Here's how the part is built. I have some questions about the finished solid (model axes, mm). Give positions to 0.01 mm unless a question says otherwise; leave off trailing zeros. Loops run counter-clockwise (first coordinate to the right, second up) from the corner with the lowest first, then second, coordinate; pieces in that order, holes last. Notation, with made-up numbers: (-22.5, 83) -> (35.5, 83) arc R21 ccw to (35.5, 92) -> close; hole circle Ø11 at (66, 21.5). An arc over 180 degrees is marked (long way). Answer in a Markdown table with one row per item. Add a question column.
Item 1: For P1, Ø4, axis at x = 18, z = 11, coming from the -Y side, with a flat end and sliding along its axis, tell me the tip position at first contact or that it passes through.
Item 2: If we section it at B-B (z = 45): Write out the boundary of the cut face in (x, y).
Item 3: If I drill on line 1 (Z direction, x = 35, y = 1.3); line 2 (Z direction, x = -34.5, y = 0.9); line 3 (X direction, y = 0.75, z = 46), over which ranges is the centre line in solid material (lowest first)?
Item 4: If we section it at A-A (x = -35): Write out the boundary of the cut face in (y, z).
Item 5: We'd pull the mould along X, two halves only. Please class faces 1 (the face through (-34.675, 0.789, -43.536)), 2 (the face through (1, 0, 1)): released by +X, released by -X, zero draft, split by the parting line, or undercut.
Autodesk Inventor part; units mm, degrees
ref_plane "YZ Plane" through (0, 0, 0) normal (1, 0, 0) x (0, 1, 0)
ref_plane "XZ Plane" through (0, 0, 0) normal (0, 1, 0) x (-1, 0, 0)
ref_plane "XY Plane" through (0, 0, 0) normal (0, 0, 1) x (1, 0, 0)
sketch "Skizze1" plane through (0, 0, 0) normal (0, 1, 0) x (-1, 0, 0)
  line L0 (40, 50) -> (-40, 50)
  line L1 (-40, 50) -> (-40, -50)
  line L2 (-40, -50) -> (40, -50)
  line L3 (40, -50) -> (40, 50)
  line L4 (0, 0) -> (0, -50) construction
  line L5 (0, 0) -> (40, 0) construction
  line L6 (35, 45) -> (-35, 45) construction
  line L7 (-35, 45) -> (-35, -45) construction
  line L8 (-35, -45) -> (35, -45) construction
  line L9 (35, -45) -> (35, 45) construction
  circle A0 centre (35, 45) radius 1.5
  circle A1 centre (-35, 45) radius 1.5
  circle A2 centre (-35, -45) radius 1.5
  circle A3 centre (35, -45) radius 1.5
  point P0 (35, 0)
  point P1 (0, -45)
  dimension "d0" = 100
  dimension "d1" = 80
  dimension "d2" = 5
  dimension "d3" = 5
  dimension "d4" = 3
  dimension "d5" = 3
  dimension "d6" = 3
  dimension "d7" = 3
extrude "Extrusion1" add sketch "Skizze1" along normal blind 1.6
properties part number "Platine_MCU"
Recorded:
| question | item | result |
|---|---|---|
| 1 | P1 | stops at y = 0 |
| 2 | outline | (-40, 0) -> (-36.5, 0) -> (-36.5, 1.6) -> (-40, 1.6) -> close; (-33.5, 0) -> (33.5, 0) -> (33.5, 1.6) -> (-33.5, 1.6) -> close; (36.5, 0) -> (40, 0) -> (40, 1.6) -> (36.5, 1.6) -> close |
| 3 | line 1 | z = -50 to -46.5, -43.5 to 43.5, 46.5 to 50 |
| 3 | line 2 | z = -50 to -46.41, -43.59 to 43.59, 46.41 to 50 |
| 3 | line 3 | x = -40 to -36.12, -33.88 to 33.88, 36.12 to 40 |
| 4 | outline | (0, -50) -> (1.6, -50) -> (1.6, -46.5) -> (0, -46.5) -> close; (0, -43.5) -> (1.6, -43.5) -> (1.6, 43.5) -> (0, 43.5) -> close; (0, 46.5) -> (1.6, 46.5) -> (1.6, 50) -> (0, 50) -> close |
| 5 | face 1 | undercut |
| 5 | face 2 | zero draft |
